```python
from build123d import *

# Parameters (mm, degrees)
BOSS_EXTRU_1_DEPTH      = 1.5
D_GAGEMENT_M41_D        = 4.3
D_GAGEMENT_M41_DEPTH    = 24
ENL_V_MAT_EXTRU_1_DEPTH = 2.5


with BuildPart() as part:
    # Esquisse1 → Boss.-Extru.1 (new body)
    with BuildSketch(Plane.XY.offset(-20)):
        Polygon((148.003126518, 65.528940229), (148.003126518, -11.471059771), (44, -11.471059771), (44, 35.528940229), (93.499999998, 35.528940229), (93.499999998, 65.528940229), align=None)
    extrude(amount=-BOSS_EXTRU_1_DEPTH)

    # Dégagement M41
    with Locations(Plane(origin=(0, 0, -21.5), x_dir=(-1, 0, 0), z_dir=(0, 0, -1))):
        with Locations((-120.751563258, 57.028940229), (-127.339384783, -2.971059771), (-64.663741735, -2.971059771)):
            Hole(D_GAGEMENT_M41_D / 2, depth=D_GAGEMENT_M41_DEPTH)

    # Esquisse5 → Enlèv. mat.-Extru.1 (cut, through all)
    with BuildSketch(Plane(origin=(0, 0, -21.5), x_dir=(-1, 0, 0), z_dir=(0, 0, -1))):
        Polygon((-97.251563258, 40.528940229), (-139.139101481, 40.528940229), (-144.251563258, 35.416478452), (-144.251563258, 18.641402007), (-139.139101481, 13.528940229), (-97.251563258, 13.528940229), align=None)
    extrude(amount=-ENL_V_MAT_EXTRU_1_DEPTH, mode=Mode.SUBTRACT)


solid = part.part
```
Geometry: final body of the model. Coordinates: model frame, mm. A direction names the side the tool comes from. Round coordinates to 2 decimals unless told otherwise and drop trailing zeros. Write each loop counter-clockwise with the first axis right and the second up, starting at its lowest first coordinate (ties: lowest second). Pieces come first, ordered by that corner, then holes. Notation, with made-up numbers: M 32,-32.75 L 72,-32.75 A32 ccw 72,-4.75 Z; hole C 83,32 d8. An arc over 180 degrees is marked long. Answer in a Markdown table with one row per item. Add a question column.
(1) Cut plane C-C, the plane x = 75.5. Return the cut outline in (y, z).
(2) Cut plane A-A, the plane y = 24. Return the cut outline in (x, z), then the cut area to 3 significant figures.
(3) Ray query, L1, parallel to Y at x = 110, z = -21.1; L2, parallel to X at y = 28.5, z = -21.2; L3, parallel to Y at x = 128.5, z = -20.1. Return the intervals inside material, ascending.
(4) Reachability of faces 1 (the face through (97, 19, -21.5)), 2 (the face through (141.73, 16.12, -20.76)) from +Z, -Z, +X, -X, +Y, -Y: full face, straight path, thin tool, end or side. Return the list, or none.
(5) Contact query for flat-ended pins moving along their axis: pin 1 (7 mm diameter, centred on x = 120.75, y = 57.03, fed in from +Z); pin 2 (0.8 mm diameter, centred on y = 45, z = -21, fed in from -X); pin 3 (10 mm diameter, centred on x = 135, y = 32, fed in from -Z) (3 decimals). Output: stop coordinate, or through.
(6) Draft query along Y for faces 3 (the face through (97, 19, -20)), 4 (the face through (62.516, -2.877, -20.74)). Return one class per face: pulls with the +Y half, pulls with the -Y half, needs draft (parallel to the pull), parting line crosses it, or undercut.
(7) Cut plane D-D, the plane y = 38. Return the cut outline in (x, z).
(8) Cut plane B-B, the plane z = -20.85. Return the cut outline in (x, y).
Established:
| question | item | result |
|---|---|---|
| 1 | outline | M -11.47,-21.5 L 35.53,-21.5 L 35.53,-20 L -11.47,-20 Z |
| 2 | outline | M 44,-21.5 L 97.25,-21.5 L 97.25,-20 L 44,-20 Z; M 144.25,-21.5 L 148,-21.5 L 148,-20 L 144.25,-20 Z |
| 2 | area | 85.5 mm² |
| 3 | L1 | -11.47 to 13.53, 40.53 to 65.53 |
| 3 | L2 | 44 to 97.25, 144.25 to 148 |
| 3 | L3 | -11.47 to -4.78, -1.16 to 13.53, 40.53 to 65.53 |
| 4 | face 1 | -Z, +X, -X, +Y, -Y |
| 4 | face 2 | +Z, -Z |
| 5 | pin 1 | z = -20 |
| 5 | pin 2 | x = 93.5 |
| 5 | pin 3 | through |
| 6 | face 3 | needs draft |
| 6 | face 4 | undercut |
| 7 | outline | M 93.5,-21.5 L 97.25,-21.5 L 97.25,-20 L 93.5,-20 Z; M 141.67,-21.5 L 148,-21.5 L 148,-20 L 141.67,-20 Z |
| 8 | outline | M 44,-11.47 L 148,-11.47 L 148,65.53 L 93.5,65.53 L 93.5,35.53 L 44,35.53 Z; hole C 64.66,-2.97 d4.3; hole M 97.25,13.53 L 139.14,13.53 L 144.25,18.64 L 144.25,35.42 L 139.14,40.53 L 97.25,40.53 Z; hole C 120.75,57.03 d4.3; hole C 127.34,-2.97 d4.3 |
